Here's how the part is built. I have some questions about the finished solid (model axes, mm). Face numbers are marked on the shaded views. A direction names the side the tool comes from. Give positions to 0.01 mm unless a question says otherwise; leave off trailing zeros. Write each loop counter-clockwise with the first axis right and the second up, starting at its lowest first coordinate (ties: lowest second). Pieces come first, ordered by that corner, then holes. Notation, with made-up numbers: (82, 83) - (128, 83) arc R35 cw to (128, 121) - close; hole circle Ø2 at (66, -26). An arc over 180 degrees is marked (long way). Use a Markdown table: item, result.
```python
from build123d import *

# Parameters (mm, degrees)
SKETCH1_R               = 50.8
BOSS_EXTRUDE1_DEPTH     = 25.4
CUT_EXTRUDE_THIN2_START = -12.7
SKETCH23_R              = 50.8
SKETCH23_R_2            = 47.625
CUT_EXTRUDE_THIN2_DEPTH = 12.7
SKETCH26_R              = 57.206394865
BOSS_EXTRUDE3_DEPTH     = 6.35
SKETCH31_R              = 48.307957565
BOSS_EXTRUDE4_DEPTH     = 2.54
SKETCH32_R              = 50.900583186
BOSS_EXTRUDE5_DEPTH     = 10.16
CUT_EXTRUDE5_DEPTH      = 85.795655708
CUT_EXTRUDE5_DEPTH_BACK = 85.795655708
SKETCH20_R              = 17.4625
CUT_EXTRUDE6_DEPTH      = 85.795655708
CUT_EXTRUDE6_DEPTH_BACK = 85.795655708
SKETCH21_R              = 8.5725


with BuildPart() as part:
    # Sketch1 → Boss-Extrude1 (new body)
    with BuildSketch(Plane.XY):
        Circle(SKETCH1_R)
    extrude(amount=BOSS_EXTRUDE1_DEPTH)

    # Sketch23 → Cut-Extrude-Thin2 (cut)
    with BuildSketch(Plane.XY.offset(25.4).offset(CUT_EXTRUDE_THIN2_START)):
        Circle(SKETCH23_R)
        Circle(SKETCH23_R_2, mode=Mode.SUBTRACT)
    extrude(amount=CUT_EXTRUDE_THIN2_DEPTH, mode=Mode.SUBTRACT)

    # Sketch26 → Boss-Extrude3 (add)
    with BuildSketch(Plane.XY.offset(12.7)):
        Circle(SKETCH26_R)
    extrude(amount=-BOSS_EXTRUDE3_DEPTH)

    # Sketch31 → Boss-Extrude4 (add)
    with BuildSketch(Plane(origin=(0, 0, 0), x_dir=(-1, 0, 0), z_dir=(0, 0, -1))):
        Circle(SKETCH31_R)
    extrude(amount=BOSS_EXTRUDE4_DEPTH)

    # Sketch32 → Boss-Extrude5 (add)
    with BuildSketch(Plane(origin=(0, 0, -2.54), x_dir=(-1, 0, 0), z_dir=(0, 0, -1))):
        Circle(SKETCH32_R)
    extrude(amount=BOSS_EXTRUDE5_DEPTH)

    # Sketch20 → Cut-Extrude5 (cut, two sides: drawn at the far end of the back side and taken through both)
    with BuildSketch(Plane(origin=(0, 0, 0), x_dir=(-1, 0, 0), z_dir=(0, 0, -1)).offset(-CUT_EXTRUDE5_DEPTH_BACK)):
        with Locations((0, 15.24)):
            Circle(SKETCH20_R)
    extrude(amount=CUT_EXTRUDE5_DEPTH + CUT_EXTRUDE5_DEPTH_BACK, mode=Mode.SUBTRACT)

    # Sketch21 → Cut-Extrude6 (cut, two sides: drawn at the far end of the back side and taken through both)
    with BuildSketch(Plane(origin=(0, 0, 0), x_dir=(-1, 0, 0), z_dir=(0, 0, -1)).offset(-CUT_EXTRUDE6_DEPTH_BACK)):
        with Locations((0, -31.086483225)):
            Circle(SKETCH21_R)
    extrude(amount=CUT_EXTRUDE6_DEPTH + CUT_EXTRUDE6_DEPTH_BACK, mode=Mode.SUBTRACT)


solid = part.part
```
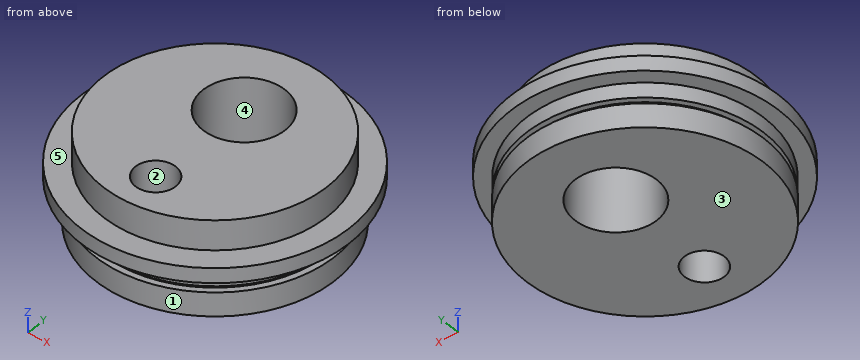
Item 1: If we section it at C-C, the plane x = 15: Write out the boundary of the cut face in (y, z).
Values:
| item | result |
|---|---|
| outline | (-55.2, 6.35) - (-48.53, 6.35) - (-48.53, 0) - (-45.92, 0) - (-45.92, -2.54) - (-48.64, -2.54) - (-48.64, -12.7) - (6.3, -12.7) - (6.3, 25.4) - (-45.2, 25.4) - (-45.2, 12.7) - (-55.2, 12.7) - close; (24.18, -12.7) - (48.64, -12.7) - (48.64, -2.54) - (45.92, -2.54) - (45.92, 0) - (48.53, 0) - (48.53, 6.35) - (55.2, 6.35) - (55.2, 12.7) - (45.2, 12.7) - (45.2, 25.4) - (24.18, 25.4) - close |
Item 2: If we section it at A-A, the plane y = 6: Write out the boundary of the cut face in (x, z).
Values:
| item | result |
|---|---|
| outline | (-56.89, 6.35) - (-50.44, 6.35) - (-50.44, 0) - (-47.93, 0) - (-47.93, -2.54) - (-50.55, -2.54) - (-50.55, -12.7) - (-14.82, -12.7) - (-14.82, 25.4) - (-47.25, 25.4) - (-47.25, 12.7) - (-56.89, 12.7) - close; (14.82, -12.7) - (50.55, -12.7) - (50.55, -2.54) - (47.93, -2.54) - (47.93, 0) - (50.44, 0) - (50.44, 6.35) - (56.89, 6.35) - (56.89, 12.7) - (47.25, 12.7) - (47.25, 25.4) - (14.82, 25.4) - close |
Item 3: Will these pins go through, and if not, where does the flat tip stop? pin 1 Ø4 at (x, z) = (-34, 15) entering from -Y; pin 2 Ø8 at (y, z) = (-5, -7.5) entering from -X; pin 3 Ø1.5 at (y, z) = (-37.5, -2.5) entering from -X.
Values:
| item | result |
|---|---|
| pin 1 | stops at y = -35.27 |
| pin 2 | stops at x = -50.89 |
| pin 3 | stops at x = -35.22 |
Item 4: For the marked faces 4 and 5, which set-ups out of +Z, -Z, +X, -X, +Y, -Y let a thin tool reach every point of the face, with its end or its side?
Values:
| item | result |
|---|---|
| face 4 | +Z, -Z |
| face 5 | +Z |
Item 5: If we section it at B-B, the plane x = 0: Count the separate pieces of the cut face and the enclosed holes in it, plus the area to 3 significant figures.
Values:
| item | result |
|---|---|
| separate pieces | 3 |
| enclosed holes | 0 |
| area | 1,880 mm2 |
Item 6: I need wall thicknesses on line 1 along Y through (x, z) = (0, -2.5); line 2 along Y through (x, z) = (0, 16) (1 decimal); line 3 along X through (y, z) = (-29, 13.5). Which ranges of each line are inside material? Lowest first, please. Write a range as [from, to].
Values:
| item | result |
|---|---|
| line 1 | y = [-48.31, -39.66], [-22.51, -2.22], [32.7, 48.31] |
| line 2 | y = [-47.6, -39.7], [-22.5, -2.2], [32.7, 47.6] |
| line 3 | x = [-37.78, -8.31], [8.31, 37.78] |
Item 7: Thinking about a two-plate mould opening in Y: for the marked faces 1, 2 and 3, which applies, +Y half, -Y half, draft (parallel to the pull), parting line (faces both ways), or undercut?
Values:
| item | result |
|---|---|
| face 1 | parting line |
| face 2 | undercut |
| face 3 | draft |
Item 8: If we section it at D-D, the plane z = 10: Write out the boundary of the cut face in (x, y) (1 decimal), plus the area to 3 significant figures.
Values:
| item | result |
|---|---|
| outline | circle Ø114.4 at (0, 0); hole circle Ø34.9 at (0, 15.2); hole circle Ø17.1 at (0, -31.1) |
| area | 9,090 mm2 |
